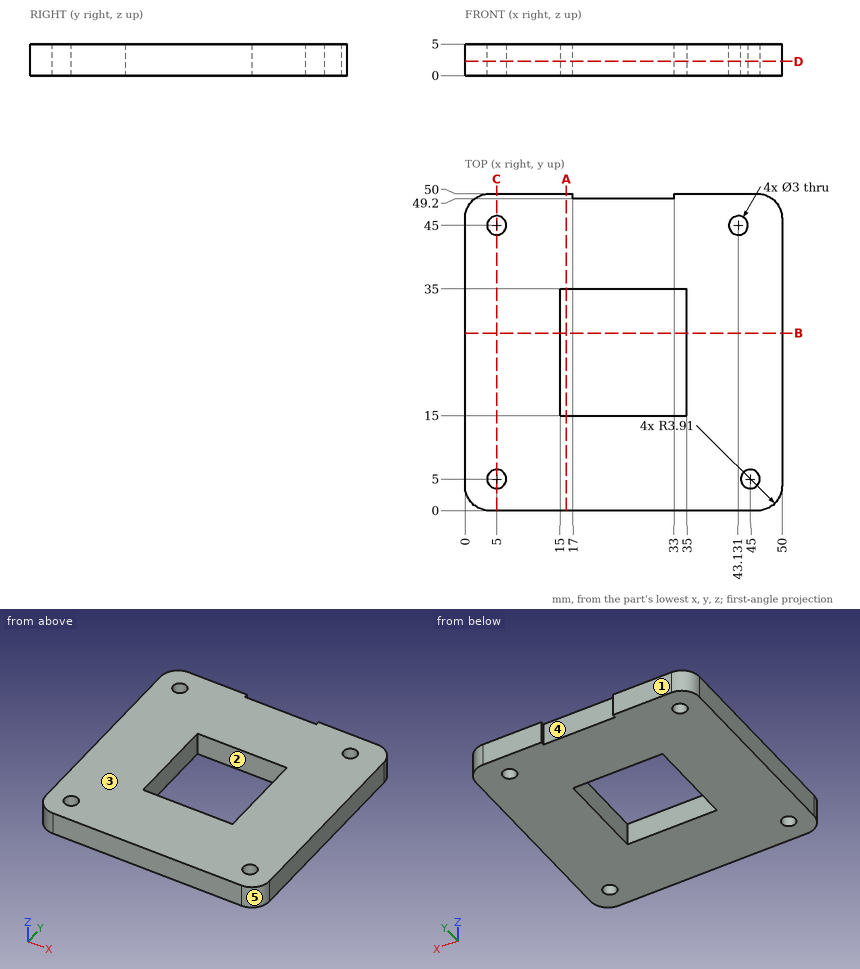
Source: three-view drawing plus pictorial views. Frame: mm from the lowest corner of the part. A direction names the side the tool comes from. Round coordinates to 2 decimals unless told otherwise and drop trailing zeros. Order: outer loops, then holes, each group sorted by start corner. A loop starts at its lowest first (then second) coordinate and runs counter-clockwise, first axis right, second up. Notation, with made-up numbers: (54.5, 71.25) -> (110.5, 71.25) arc R7 cw to (110.5, 84.25) -> close; hole circle Ø1 at (40.5, 34.25). An arc over 180 degrees is marked (long way). Use CSV: the item, a comma, the result in double quotes. Start each with the question number.
1) Set-up query: the marked faces 1 and 2. Return all of +Z, -Z, +X, -X, +Y, -Y with unobstructed straight access to the full face (end or side cutting, diameter ignored); none if empty.
2) Section A-A (x = 16). Return the cut outline in (y, z).
3) Section D-D (z = 2.25). Return the cut outline in (x, y), and give its area (3 significant figures).
4) First-contact query: pin 1 Ø3 at (x, z) = (15.5, 0.5) entering from -Y. Flat tip, straight axial feed; report the tip coordinate or a pass-through.
5) Material intervals for line 1 along Y through (x, z) = (5, 2.9); line 2 along Y through (x, z) = (20.5, 2.4); line 3 along Y through (x, z) = (6, 1.4), sorted ascending. Write a range as from..to.
6) Section C-C (x = 5). Return the cut outline in (y, z), and give its area (3 significant figures).
7) Draft query along X for the marked faces 3, 4 and 5. Return one class per face: +X half, -X half, draft (parallel to the pull), parting line (faces both ways), or undercut.
Returned:
1,face 1,"+Z, -Z, +X, -X, +Y"
1,face 2,"+Z, -Z"
2,outline,"(0, 0) -> (15, 0) -> (15, 5) -> (0, 5) -> close; (35, 0) -> (50, 0) -> (50, 5) -> (35, 5) -> close"
3,outline,"(0, 3.91) arc R3.91 ccw to (3.91, 0) -> (46.09, 0) arc R3.91 ccw to (50, 3.91) -> (50, 46.09) arc R3.91 ccw to (46.09, 50) -> (33, 50) -> (33, 49.2) -> (17, 49.2) -> (17, 50) -> (3.91, 50) arc R3.91 ccw to (0, 46.09) -> close; hole circle Ø3 at (5, 5); hole circle Ø3 at (5, 45); hole (15, 15) -> (35, 15) -> (35, 35) -> (15, 35) -> close; hole circle Ø3 at (43.13, 45); hole circle Ø3 at (45, 5)"
3,area,"2,050 mm²"
4,pin 1,"stops at y = 0"
5,line 1,"y = 0..3.5, 6.5..43.5, 46.5..50"
5,line 2,"y = 0..15, 35..49.2"
5,line 3,"y = 0..3.88, 6.12..43.88, 46.12..50"
6,outline,"(0, 0) -> (3.5, 0) -> (3.5, 5) -> (0, 5) -> close; (6.5, 0) -> (43.5, 0) -> (43.5, 5) -> (6.5, 5) -> close; (46.5, 0) -> (50, 0) -> (50, 5) -> (46.5, 5) -> close"
6,area,"220 mm²"
7,face 3,"draft"
7,face 4,"undercut"
7,face 5,"+X half"
